```python
from build123d import *

# Parameters (mm, degrees)
BOSS_EXTRUDE1_DEPTH = 35
CUT_EXTRUDE1_REACH  = 119.154
CUT_EXTRUDE2_REACH  = 119.154
SKETCH3_R           = 2
CUT_EXTRUDE3_REACH  = 119.154
SKETCH4_R           = 2


with BuildPart() as part:
    # Sketch1 → Boss-Extrude1 (new body)
    with BuildSketch(Plane.XY):
        Polygon((0, 0), (-50, 0), (-50, 100), (0, 100), (0, 97), (-47, 97), (-47, 3), (0, 3), align=None)
    extrude(amount=BOSS_EXTRUDE1_DEPTH)

    # Sketch2 → Cut-Extrude1 (cut, up to next)
    with BuildSketch(Plane.XZ, mode=Mode.PRIVATE) as cut_extrude1_sk1:
        with BuildLine():
            Line((0, 13.4), (-24, 13.4))
            ThreePointArc((-24, 13.4), (-28.1, 17.5), (-24, 21.6))
            Line((-24, 21.6), (0, 21.6))
            Line((0, 21.6), (0, 13.4))
        make_face()
    cut_extrude1_tool1 = extrude(cut_extrude1_sk1.sketch, amount=-CUT_EXTRUDE1_REACH, mode=Mode.PRIVATE) & part.part
    add(cut_extrude1_tool1.solids().sort_by_distance((-13.625448, 0, 17.5))[0], mode=Mode.SUBTRACT)

    # Sketch3 → Cut-Extrude2 (cut, up to next)
    with BuildSketch(Plane(origin=(0, 100, 0), x_dir=(1, 0, 0), z_dir=(0, 1, 0)), mode=Mode.PRIVATE) as cut_extrude2_sk1:
        with Locations(Location((-22, -10, 0), (0, 0, 270))):
            Circle(SKETCH3_R)
    cut_extrude2_tool1 = extrude(cut_extrude2_sk1.sketch, amount=-CUT_EXTRUDE2_REACH, mode=Mode.PRIVATE) & part.part
    # Sketch3 → Cut-Extrude2 (cut, up to next)
    with BuildSketch(Plane(origin=(0, 100, 0), x_dir=(1, 0, 0), z_dir=(0, 1, 0)), mode=Mode.PRIVATE) as cut_extrude2_sk2:
        with Locations(Location((-10, -10, 0), (0, 0, 270))):
            Circle(SKETCH3_R)
    cut_extrude2_tool2 = extrude(cut_extrude2_sk2.sketch, amount=-CUT_EXTRUDE2_REACH, mode=Mode.PRIVATE) & part.part
    add(cut_extrude2_tool1.solids().sort_by_distance((-22, 100, 10))[0], mode=Mode.SUBTRACT)
    add(cut_extrude2_tool2.solids().sort_by_distance((-10, 100, 10))[0], mode=Mode.SUBTRACT)

    # Sketch4 → Cut-Extrude3 (cut, up to next)
    with BuildSketch(Plane.ZY.offset(50), mode=Mode.PRIVATE) as cut_extrude3_sk1:
        with Locations((17.5, 60)):
            Circle(SKETCH4_R)
    cut_extrude3_tool1 = extrude(cut_extrude3_sk1.sketch, amount=-CUT_EXTRUDE3_REACH, mode=Mode.PRIVATE) & part.part
    # Sketch4 → Cut-Extrude3 (cut, up to next)
    with BuildSketch(Plane.ZY.offset(50), mode=Mode.PRIVATE) as cut_extrude3_sk2:
        with Locations((17.5, 40)):
            Circle(SKETCH4_R)
    cut_extrude3_tool2 = extrude(cut_extrude3_sk2.sketch, amount=-CUT_EXTRUDE3_REACH, mode=Mode.PRIVATE) & part.part
    add(cut_extrude3_tool1.solids().sort_by_distance((-50, 60, 17.5))[0], mode=Mode.SUBTRACT)
    add(cut_extrude3_tool2.solids().sort_by_distance((-50, 40, 17.5))[0], mode=Mode.SUBTRACT)


solid = part.part
```
The model under review builds one solid part; all positions refer to its coordinate system, in mm. A direction names the side the tool comes from. Round coordinates to 2 decimals unless told otherwise and drop trailing zeros. Loops run counter-clockwise (first coordinate to the right, second up) from the corner with the lowest first, then second, coordinate; pieces in that order, holes last. Notation, with made-up numbers: (82, 23.25) - (127, 23.25) arc R25 ccw to (127, 61.25) - close; hole circle Ø6 at (22.25, -16.75). An arc over 180 degrees is marked (long way). Write each question's results on one line, items separated by ' | '. Start each with the question number.
Q1. Draft analysis for pull direction X (two halves, no side actions). For faces 1 (the cylindrical face through (-20, 99, 10)), 2 (the flat face through (-49, 50, 35)), 3 (the cylindrical face through (-8, 99, 10)), 4 (the flat face through (-50, 49, 17)), state which applies: pulls with the +X half, pulls with the -X half, needs draft (parallel to the pull), parting line crosses it, or undercut.
Q2. Insertion check: P1, Ø10, axis at y = 74, z = 17, coming from the +X side. The pin has a flat end and moves straight along its axis. Give the tip position at first contact, or say it passes through.
Q3. Take a section at C-C on x = -15. Give the boundary of the cut face in (y, z), plus the area to 3 significant figures.
Q4. Take a section at B-B on z = 10. Give the boundary of the cut face in (x, y), plus the area to 3 significant figures.
Q5. Tool access review of faces 5 (the cylindrical face through (-48.521, 61.983, 17.24)), 6 (the cylindrical face through (-28.1, 1.5, 17.4)), 7 (the flat face through (-23, 97, 17)): name each direction out of +Z, -Z, +X, -X, +Y, -Y from which nothing blocks a thin tool from reaching the whole face with its end or side.
Q6. Wall thickness on line 1 along X through (y, z) = (99, 10); line 2 along Y through (x, z) = (-48.65, 17.5); line 3 along Y through (x, z) = (-28, 12.5): over which ranges is each line inside the solid? List them lowest first. Write a range as [from, to].
Q7. Take a section at A-A on x = -35.5. Give the boundary of the cut face in (y, z).
Q8. Take a section at D-D on x = -22. Give the boundary of the cut face in (y, z).
Data:
1) face 1: undercut | face 2: needs draft | face 3: undercut | face 4: pulls with the -X half
2) P1: stops at x = -47
3) outline: (0, 0) - (3, 0) - (3, 13.4) - (0, 13.4) - close; (0, 21.6) - (3, 21.6) - (3, 35) - (0, 35) - close; (97, 0) - (100, 0) - (100, 35) - (97, 35) - close | area: 185 mm²
4) outline: (-50, 0) - (0, 0) - (0, 3) - (-47, 3) - (-47, 97) - (-24, 97) - (-24, 100) - (-50, 100) - close; (-20, 97) - (-12, 97) - (-12, 100) - (-20, 100) - close; (-8, 97) - (0, 97) - (0, 100) - (-8, 100) - close | area: 558 mm²
5) face 5: +X, -X | face 6: +X, -Y | face 7: +Z, -Z, +X
6) line 1: x = [-50, -24], [-20, -12], [-8, 0] | line 2: y = [0, 38], [42, 58], [62, 100] | line 3: y = [0, 3], [97, 100]
7) outline: (0, 0) - (3, 0) - (3, 35) - (0, 35) - close; (97, 0) - (100, 0) - (100, 35) - (97, 35) - close
8) outline: (0, 0) - (3, 0) - (3, 13.4) - (0, 13.4) - close; (0, 21.6) - (3, 21.6) - (3, 35) - (0, 35) - close; (97, 0) - (100, 0) - (100, 8) - (97, 8) - close; (97, 12) - (100, 12) - (100, 35) - (97, 35) - close
